Read the model definition and answer for the solid it produces. Units are mm, in the model's axes. Face numbers are marked on the shaded views. Round coordinates to 2 decimals unless told otherwise and drop trailing zeros. Loops run counter-clockwise (first coordinate to the right, second up) from the corner with the lowest first, then second, coordinate; pieces in that order, holes last. Notation, with made-up numbers: (1.25, 66.25) - (17.25, 66.25) arc R20 cw to (17.25, 95.25) - close; hole circle Ø11 at (-17.75, 36.5). An arc over 180 degrees is marked (long way). Answer as CSV lines item,"result".
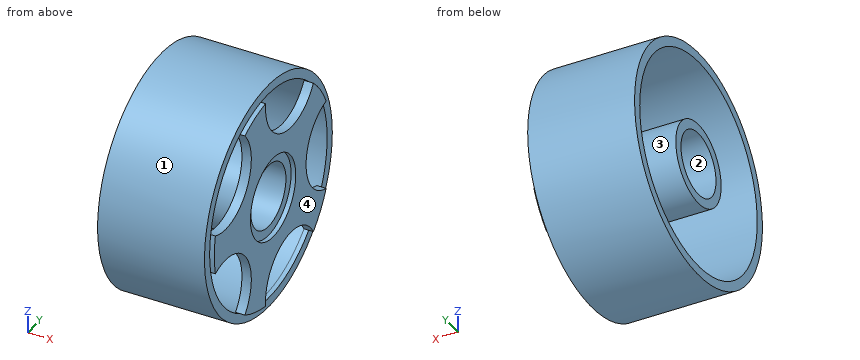
Autodesk Inventor part; units mm, degrees
ref_plane "YZ Plane" through (0, 0, 0) normal (1, 0, 0) x (0, 1, 0)
ref_plane "XZ Plane" through (0, 0, 0) normal (0, 1, 0) x (-1, 0, 0)
ref_plane "XY Plane" through (0, 0, 0) normal (0, 0, 1) x (1, 0, 0)
sketch "Sketch1" plane through (0, 0, 0) normal (1, 0, 0) x (0, 1, 0)
  circle A0 centre (11.1737, 22.3473) radius 5.588
  circle A1 centre (11.1737, 22.3473) radius 4.318
  circle A2 centre (11.1737, 22.3473) radius 14.478
  circle A3 centre (11.1737, 22.3473) radius 15.748
  point P0 (0, 0)
  dimension "d0" = 11.176
  dimension "d1" = 1.27
  dimension "d2" = 1.27
  dimension "d3" = 8.89
extrude "Extrusion1" add sketch "Sketch1" against normal blind 14.478 contours A3
extrude "Extrusion2" add sketch "Sketch1" against normal blind 14.478 contours A0
sketch "Sketch2" plane through (0, 11.1737, 22.3473) normal (1, 0, 0) x (0, 0, -1)
  circle A0 centre (0, 0) radius 14.478
  circle A1 centre (0, 0) radius 15.748
  circle A2 centre (0, 0) radius 5.588
  circle A3 centre (0, 0) radius 4.318
  point P0 (22.3473, -11.1737)
extrude "Extrusion3" add sketch "Sketch2" along normal mid plane 1.27 contours A0
sketch "Sketch3" plane through (0.635, 11.1737, 22.3473) normal (1, 0, 0) x (0, 0, -1)
  circle A0 centre (0, 0) radius 14.478
  arc A1 (-6.1954, 13.0855) -> (6.1954, 13.0855) centre (0, 14.478) ccw
  arc A2 (6.1954, 13.0855) -> (-6.1954, 13.0855) centre (0, 0) ccw
  arc A3 (-14.3595, -1.8486) -> (-10.5305, 9.9358) centre (-13.7694, 4.4739) ccw
  arc A4 (-10.5305, 9.9358) -> (-14.3595, -1.8486) centre (0, 0) ccw
  arc A5 (-2.6792, -14.2279) -> (-12.7036, -6.9448) centre (-8.51, -11.7129) ccw
  arc A6 (-12.7036, -6.9448) -> (-2.6792, -14.2279) centre (0, 0) ccw
  arc A7 (12.7036, -6.9448) -> (2.6792, -14.2279) centre (8.51, -11.7129) ccw
  arc A8 (2.6792, -14.2279) -> (12.7036, -6.9448) centre (0, 0) ccw
  arc A9 (10.5305, 9.9358) -> (14.3595, -1.8486) centre (13.7694, 4.4739) ccw
  arc A10 (14.3595, -1.8486) -> (10.5305, 9.9358) centre (0, 0) ccw
  point P0 (22.3473, -11.1737)
  dimension "d10" = 12.7
  dimension "d13" = 360
extrude "Extrusion4" cut sketch "Sketch3" against normal up to next contours A0 A9 | A1 A0 | A0 A7 | A3 A0 | A0 A5
properties part number "wheal"
1) A cutting plane is placed at B-B, the plane x = -9. Determine the outline of the cut face in (y, z), plus the area to 3 significant figures.
Entries:
outline,"circle Ø31.5 at (11.17, 22.35); circle Ø11.18 at (11.17, 22.35); hole circle Ø28.96 at (11.17, 22.35); hole circle Ø8.64 at (11.17, 22.35)"
area,"160 mm^2"
2) Find the intervals of material crossed by line 1 (Z direction, x = -7.5, y = 16); line 2 (Y direction, x = -8.25, z = 22); line 3 (Y direction, x = -2.5, z = 27.5), in increasing order.
Entries:
line 1,"z = 7.36 to 8.7, 19.53 to 25.16, 36 to 37.34"
line 2,"y = -4.57 to -3.3, 5.6 to 6.87, 15.48 to 16.75, 25.65 to 26.92"
line 3,"y = -3.71 to -2.36, 9.01 to 13.34, 24.7 to 26.05"
3) A cutting plane is placed at C-C, the plane y = 22.5. Determine the outline of the cut face in (x, z) (3 decimals), plus the area to 3 significant figures.
Entries:
outline,"(-14.478, 11.406) - (0, 11.406) - (0, 13.329) - (0.635, 13.329) - (0.635, 16.835) - (-0.635, 16.835) - (-0.635, 13.329) - (-14.478, 13.329) - close; (-14.478, 31.365) - (-0.635, 31.365) - (-0.635, 27.86) - (0.635, 27.86) - (0.635, 31.365) - (0, 31.365) - (0, 33.289) - (-14.478, 33.289) - close"
area,"64.6 mm^2"
4) A cutting plane is placed at D-D, the plane y = 5. Determine the outline of the cut face in (x, z) (3 decimals).
Entries:
outline,"(-14.478, 7.86) - (0, 7.86) - (0, 9.252) - (0.635, 9.252) - (0.635, 10.733) - (-0.635, 10.733) - (-0.635, 9.252) - (-14.478, 9.252) - close; (-14.478, 35.443) - (-0.635, 35.443) - (-0.635, 33.962) - (0.635, 33.962) - (0.635, 35.443) - (0, 35.443) - (0, 36.835) - (-14.478, 36.835) - close; (-0.635, 16.942) - (0.635, 16.942) - (0.635, 27.752) - (-0.635, 27.752) - close"
5) The mould has two halves that part along Y. Classify the marked faces 1, 2, 3 and 4: pulls with the +Y half, pulls with the -Y half, needs draft (parallel to the pull), parting line crosses it, or undercut.
Entries:
face 1,"parting line crosses it"
face 2,"undercut"
face 3,"undercut"
face 4,"needs draft"
6) Each of these flat-tipped pins is pushed along its axis until it touches: P1, Ø8, axis at y = 17, z = 14.5, coming from the -X side (3 decimals); P2, Ø12.5, axis at y = 10, z = 23, coming from the +X side (3 decimals); P3, Ø4, axis at x = -12, y = 8, coming from the +Z side; P4, Ø1.5, axis at x = -6, z = 21, coming from the +Y side. Where does it stop, or does it pass through?
Entries:
P1,"stops at x = -0.635"
P2,"stops at x = 0.635"
P3,"stops at z = 38.05"
P4,"stops at y = 26.91"
